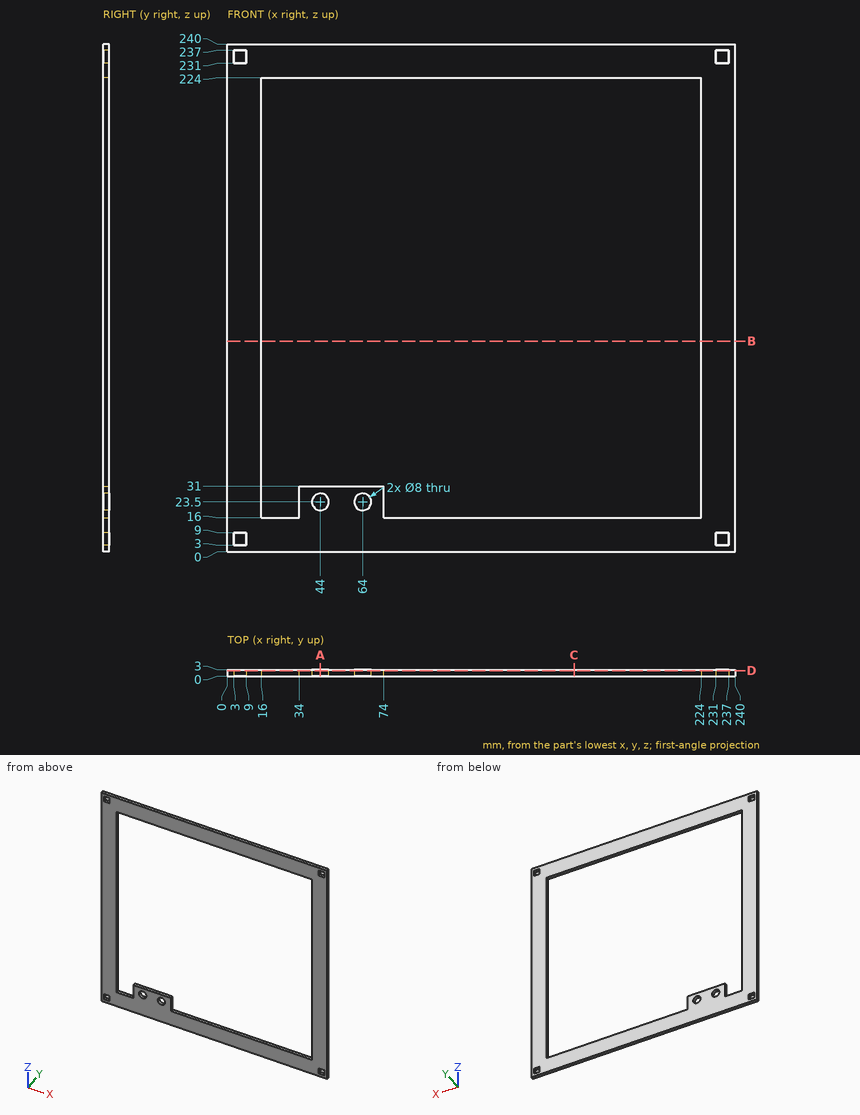
Can you work these out from the drawing? Everything is in mm from the part's minimum corner. Coordinates: 2 decimals unless noted, no trailing zeros. Write each loop counter-clockwise with the first axis right and the second up, starting at its lowest first coordinate (ties: lowest second). Pieces come first, ordered by that corner, then holes. Notation, with made-up numbers: (-35.5, -32.75) -> (14.5, -32.75) arc R26 cw to (14.5, -3.75) -> close; hole circle Ø3 at (62, 25.25). An arc over 180 degrees is marked (long way). Write each question's results on one line, items separated by ' | '. Start each with the question number.
Item 1: If we section it at B-B, the plane z = 99.5: Write out the boundary of the cut face in (x, y), and give its area (3 significant figures).
Item 2: If we section it at D-D, the plane y = 2.5: Count the separate pieces of the cut face and the enclosed holes in it, and give its area (3 significant figures).
Item 3: I'm going to push a flat-ended pin straight in: P1, Ø1.5, axis at x = 7.5, y = 1.5, coming from the -Z side. Where does the tip first touch, or does it pass through?
Item 4: If we section it at A-A, the plane x = 44: Write out the boundary of the cut face in (y, z).
Item 5: Please list where these lines run through material, in increasing order: probe 1 along Z at (x, y) = (64, 0.85); probe 2 along Z at (x, y) = (57, 2.25); probe 3 along X at (y, z) = (2.35, 115).
Item 6: If we section it at C-C, the plane x = 164: Write out the boundary of the cut face in (y, z).
Answer block:
1) outline: (0, 0) -> (16, 0) -> (16, 3) -> (0, 3) -> close; (224, 0) -> (240, 0) -> (240, 3) -> (224, 3) -> close | area: 96.0 mm²
2) separate pieces: 1 | enclosed holes: 7 | area: 14,700 mm²
3) P1: z = 0
4) outline: (0, 0) -> (3, 0) -> (3, 19.5) -> (0, 19.5) -> close; (0, 27.5) -> (3, 27.5) -> (3, 31) -> (0, 31) -> close; (0, 224) -> (3, 224) -> (3, 240) -> (0, 240) -> close
5) probe 1: 0 to 19.5, 27.5 to 31, 224 to 240 | probe 2: 0 to 31, 224 to 240 | probe 3: 0 to 16, 224 to 240
6) outline: (0, 0) -> (3, 0) -> (3, 16) -> (0, 16) -> close; (0, 224) -> (3, 224) -> (3, 240) -> (0, 240) -> close
